from build123d import *

# Parameters (mm, degrees)
F0_W     = 139.7
F0_H     = 127
F1_DEPTH = 19.05
F2_R     = 7.62
F3_R     = 7.62


with BuildPart() as f1:
    # F0 (on Front) → F1 (new body)
    with BuildSketch(Plane.XZ):
        Rectangle(F0_W, F0_H)
    extrude(amount=F1_DEPTH)

    # F2
    f2_edges = [f1.edges().sort_by_distance(p)[0] for p in [
        (69.85, 0, 0),
        (0, 0, -63.5),
    ]]
    fillet(f2_edges, radius=F2_R)

    # F3
    f3_edges = [f1.edges().sort_by_distance(p)[0] for p in [
        (-69.85, 0, 3.81),
    ]]
    fillet(f3_edges, radius=F3_R)


solid = f1.part
The model under review builds one solid part; all positions refer to its coordinate system, in mm. Round coordinates to 2 decimals unless told otherwise and drop trailing zeros. Order: outer loops, then holes, each group sorted by start corner. A loop starts at its lowest first (then second) coordinate and runs counter-clockwise, first axis right, second up. Notation, with made-up numbers: (67.5, 87.5) -> (87.5, 87.5) arc R18 ccw to (87.5, 117.5) -> close; hole circle Ø2 at (-6, 79.5). An arc over 180 degrees is marked (long way). Write item = value, one per line. Start each with the question number.
Item 1: For line 1 along X through (y, z) = (-7, 54.5); line 2 along X through (y, z) = (-4.25, 18.5); line 3 along Z through (x, y) = (-28.5, -3.5), list the stretches that pass through material, from the lowest coordinate up.
Item 2: Clearance check with flat-ended pins moving along their axes: pin 1 Ø1 at (y, z) = (-5, -34.5) entering from +X; pin 2 Ø3 at (x, y) = (-22.5, -5.5) entering from -Z; pin 3 Ø10 at (y, z) = (-4.5, 32) entering from -X. State where each tip first meets the part, or that it passes through.
Item 3: Consider section A-A on y = -2.25. Write out the cut boundary in (x, z), plus the area to 3 significant figures.
Conclusion:
q1.line_1 = -69.82 to 69.82
q1.line_2 = -69.06 to 69.06
q1.line_3 = -62.29 to 63.5
q2.pin_1 = 69.55
q2.pin_2 = -63.47
q2.pin_3 = -69.85
q3.outline = (-67.64, -55.88) arc R5.41 ccw to (-62.23, -61.29) -> (67.64, -61.29) -> (67.64, 63.5) -> (-67.64, 63.5) -> close
q3.area = 16,900 mm2
